Part model, mm, in its own coordinate system. Face numbers are marked on the shaded views. A direction names the side the tool comes from. Coordinates: 2 decimals unless noted, no trailing zeros. Order: outer loops, then holes, each group sorted by start corner. A loop starts at its lowest first (then second) coordinate and runs counter-clockwise, first axis right, second up.
from build123d import *

# Parameters (mm, degrees)
SKETCH_1_W          = 29.5
SKETCH_1_H          = 29
EXTRUDE_1_DEPTH     = 7
SKETCH_2_W          = 5
SKETCH_2_H          = 14
EXTRUDE_2_DEPTH     = 2
SKETCH_3_R          = 2.25
CUT_EXTRUDE_1_DEPTH = 35.176929353
SKETCH_4_R          = 6.5
SKETCH_4_R_2        = 2.5
EXTRUDE_3_DEPTH     = 5
SKETCH_5_R          = 3
EXTRUDE_4_DEPTH     = 3.5
EXTRUDE_START       = 10
SKETCH_4_3_R        = 10.5
EXTRUDE_5_DEPTH     = 2
SKETCH_4_4_R        = 2.5
EXTRUDE_6_DEPTH     = 10
CUT_EXTRUDE_2_REACH = 51.805
SKETCH_6_R          = 1


with BuildPart() as part:
    # Sketch 1 → Extrude 1 (new, symmetric)
    with BuildSketch(Plane.XY):
        with Locations((0, -14.5)):
            Rectangle(SKETCH_1_W, SKETCH_1_H)
    extrude(amount=EXTRUDE_1_DEPTH, both=True)

    # Sketch 2 → Extrude 2 (add)
    with BuildSketch(Plane(origin=(0, -2, 0), x_dir=(1, 0, 0), z_dir=(0, 1, 0))):
        with Locations((17.25, 0)):
            Rectangle(SKETCH_2_W, SKETCH_2_H)
    extrude_2 = extrude(amount=-EXTRUDE_2_DEPTH)

    # Sketch 3 → Cut-Extrude 1 (cut, through all)
    with BuildSketch(Plane(origin=(0, -2, 0), x_dir=(1, 0, 0), z_dir=(0, 1, 0))):
        with Locations((18, 0)):
            Circle(SKETCH_3_R)
    cut_extrude_1 = extrude(amount=-CUT_EXTRUDE_1_DEPTH, mode=Mode.SUBTRACT)

    # Sketch 4 → Extrude 3 (add)
    with BuildSketch(Plane(origin=(0, 0, 0), x_dir=(1, 0, 0), z_dir=(0, 1, 0))):
        with Locations(Location((7.25, 0, 0), (0, 0, 270))):
            Circle(SKETCH_4_R)
        with Locations(Location((7.25, 0, 0), (0, 0, 270))):
            Circle(SKETCH_4_R_2, mode=Mode.SUBTRACT)
    extrude(amount=EXTRUDE_3_DEPTH)

    # Mirror 1: Extrude 2, Cut-Extrude 1 across plane
    add(extrude_2.mirror(Plane(origin=(0, 0, 0), x_dir=(0, 0, 1), z_dir=(1, 0, 0))))
    add(cut_extrude_1.mirror(Plane(origin=(0, 0, 0), x_dir=(0, 0, 1), z_dir=(1, 0, 0))), mode=Mode.SUBTRACT)

    # Sketch 5 → Extrude 4 (add)
    with BuildSketch(Plane.XZ.offset(29)):
        with Locations(Location((8.75, 0, 0), (0, 0, 180))):
            Circle(SKETCH_5_R)
    extrude(amount=EXTRUDE_4_DEPTH)



with BuildPart() as body_2:
    # Sketch 4_3 → Extrude 5 (new body)
    with BuildSketch(Plane(origin=(0, 0, 0), x_dir=(1, 0, 0), z_dir=(0, 1, 0)).offset(EXTRUDE_START)):
        with Locations(Location((7.25, 0, 0), (0, 0, 270))):
            Circle(SKETCH_4_3_R)
    extrude(amount=EXTRUDE_5_DEPTH)


with BuildPart() as part_1:
    add(part.part)

    add(body_2.part)  # Extrude 6 merges body 2
    # Sketch 4_4 → Extrude 6 (add)
    with BuildSketch(Plane(origin=(0, 0, 0), x_dir=(1, 0, 0), z_dir=(0, 1, 0))):
        with Locations(Location((7.25, 0, 0), (0, 0, 270))):
            Circle(SKETCH_4_4_R)
    extrude(amount=EXTRUDE_6_DEPTH)

    # Sketch 6 → Cut-Extrude 2 (cut, up to next)
    with BuildSketch(Plane(origin=(0, 12, 0), x_dir=(1, 0, 0), z_dir=(0, 1, 0)), mode=Mode.PRIVATE) as cut_extrude_2_sk1:
        with Locations(Location((14.45, 3.3, 0), (0, 0, 270))):
            Circle(SKETCH_6_R)
    cut_extrude_2_tool1 = extrude(cut_extrude_2_sk1.sketch, amount=-CUT_EXTRUDE_2_REACH, mode=Mode.PRIVATE) & part_1.part
    # Sketch 6 → Cut-Extrude 2 (cut, up to next)
    with BuildSketch(Plane(origin=(0, 12, 0), x_dir=(1, 0, 0), z_dir=(0, 1, 0)), mode=Mode.PRIVATE) as cut_extrude_2_sk2:
        with Locations(Location((14.45, 0, 0), (0, 0, 270))):
            Circle(SKETCH_6_R)
    cut_extrude_2_tool2 = extrude(cut_extrude_2_sk2.sketch, amount=-CUT_EXTRUDE_2_REACH, mode=Mode.PRIVATE) & part_1.part
    # Sketch 6 → Cut-Extrude 2 (cut, up to next)
    with BuildSketch(Plane(origin=(0, 12, 0), x_dir=(1, 0, 0), z_dir=(0, 1, 0)), mode=Mode.PRIVATE) as cut_extrude_2_sk3:
        with Locations(Location((14.45, -3.3, 0), (0, 0, 270))):
            Circle(SKETCH_6_R)
    cut_extrude_2_tool3 = extrude(cut_extrude_2_sk3.sketch, amount=-CUT_EXTRUDE_2_REACH, mode=Mode.PRIVATE) & part_1.part
    add(cut_extrude_2_tool1.solids().sort_by_distance((14.45, 12, -3.3))[0], mode=Mode.SUBTRACT)
    add(cut_extrude_2_tool2.solids().sort_by_distance((14.45, 12, 0))[0], mode=Mode.SUBTRACT)
    add(cut_extrude_2_tool3.solids().sort_by_distance((14.45, 12, 3.3))[0], mode=Mode.SUBTRACT)


solid = part_1.part
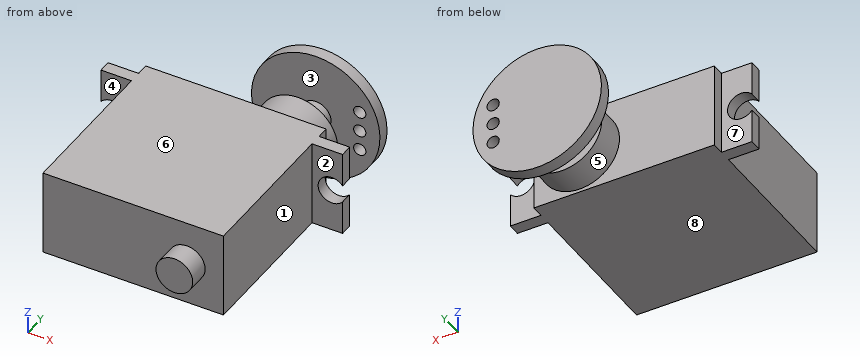
Q1. Which spindle directions (+Z, -Z, +X, -X, +Y, -Y) get a long thin tool onto all of the face, cutting with end or side? Do the marked faces 4, 5, 6, 7 and 8. Say none if no direction does.
Results list:
face 4: +Z, -Z, -X, -Y
face 5: none
face 6: +Z, +X, -X, -Y
face 7: +Z, -Z, -X, +Y
face 8: -Z, +X, -X, -Y
Q2. Cut at A-A on x = -18. Write the cut outline in (y, z).
Results list:
outline: (-4, -7) - (-2, -7) - (-2, -2.25) - (-4, -2.25) - close; (-4, 2.25) - (-2, 2.25) - (-2, 7) - (-4, 7) - close
Q3. Mould opens along Y. For the marked faces 1, 2 and 3 say: pulls with the +Y half, pulls with the -Y half, needs draft (parallel to the pull), parting line crosses it, or undercut.
Results list:
face 1: needs draft
face 2: pulls with the -Y half
face 3: undercut
Q4. Cut at B-B on z = 3.75. Write the cut outline in (x, y).
Results list:
outline: (-19.75, -4) - (-14.75, -4) - (-14.75, -29) - (14.75, -29) - (14.75, -4) - (19.75, -4) - (19.75, -2) - (14.75, -2) - (14.75, 0) - (12.56, 0) - (12.56, 5) - (1.94, 5) - (1.94, 0) - (-14.75, 0) - (-14.75, -2) - (-19.75, -2) - close; (-2.56, 10) - (13.56, 10) - (13.56, 12) - (-2.56, 12) - close; (15.34, 10) - (17.06, 10) - (17.06, 12) - (15.34, 12) - close
Q5. Cut at D-D on y = -27. Write the cut outline in (x, z), and give its area (3 significant figures).
Results list:
outline: (-14.75, -7) - (14.75, -7) - (14.75, 7) - (-14.75, 7) - close
area: 413 mm2
Q6. Wall check: line 1 along X through (y, z) = (10.6, 0); line 2 along Y through (x, z) = (8.5, 5.5); line 3 along Z through (x, y) = (14, 11). Give the ranges that are in metal, low to high.
Results list:
line 1: x = -3.25 to 13.45, 15.45 to 17.75
line 2: y = -29 to 5, 10 to 12
line 3: z = -8.04 to -4.19, -2.41 to -0.89, 0.89 to 2.41, 4.19 to 8.04
Q7. Pin check, flat tips, straight feed: pin 1 Ø4 at (y, z) = (-18, -3.5) entering from -X; pin 2 Ø14.5 at (x, y) = (0.5, -12.5) entering from -Z; pin 3 Ø11 at (y, z) = (-13, -3) entering from +X; pin 4 Ø4 at (x, z) = (-18, 0) entering from +Y. Stop position of each tip, or through.
Results list:
pin 1: stops at x = -14.75
pin 2: stops at z = -7
pin 3: stops at x = 14.75
pin 4: passes through
Q8. Cut at C-C on x = 7.25. Write the cut outline in (y, z), and give its area (3 significant figures).
Results list:
outline: (-32.5, -2.6) - (-29, -2.6) - (-29, -7) - (0, -7) - (0, -6.5) - (5, -6.5) - (5, -2.5) - (10, -2.5) - (10, -10.5) - (12, -10.5) - (12, 10.5) - (10, 10.5) - (10, 2.5) - (5, 2.5) - (5, 6.5) - (0, 6.5) - (0, 7) - (-29, 7) - (-29, 2.6) - (-32.5, 2.6) - close
area: 556 mm2
